Geometry check sheet. Reference: the model listing, model coordinates, mm. Face numbers are marked on the shaded views. A direction names the side the tool comes from. Round coordinates to 2 decimals unless told otherwise and drop trailing zeros. Order: outer loops, then holes, each group sorted by start corner. A loop starts at its lowest first (then second) coordinate and runs counter-clockwise, first axis right, second up.
(1) Material ranges on line 1 along Z through (x, y) = (-1.59, 16.65); line 2 along Z through (x, y) = (-1.2, 5.5); line 3 along Y through (x, z) = (-2.6, -7.75), recorded low to high.
(2) Set-up check for the marked faces 4, 5, 6, 7 and 8: record each of +Z, -Z, +X, -X, +Y, -Y from which the full face is reachable in a straight line by a thin tool's end or side.
(3) Go/stop test with flat-tipped pins: pin 1 (1.4 mm diameter, centred on x = -1.59, z = -8.1, fed in from -Y); pin 2 (3 mm diameter, centred on y = 11.25, z = 1.49, fed in from -X); pin 3 (1 mm diameter, centred on x = -1.5, y = 13, fed in from +Z). Record where each tip stops, or that it passes through.
(4) Release check for a two-part mould opening along Z. For the marked faces 1, 2 and 3 record: +Z half, -Z half, draft (parallel to the pull), parting line (faces both ways), or undercut.
(5) Sectioned sample at A-A (y = -18). Record the boundary of the cut face in (x, z).
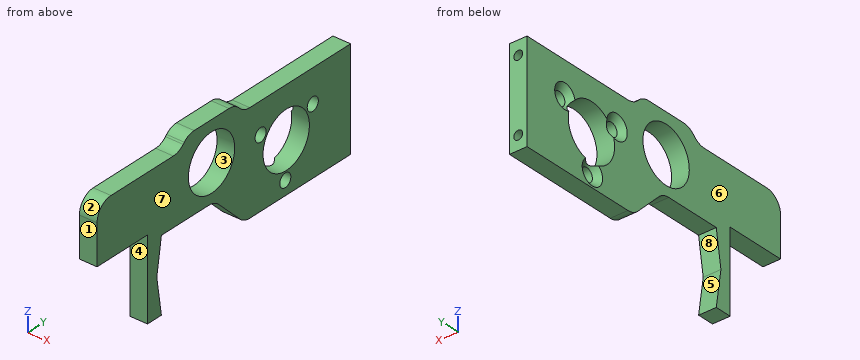
from build123d import *

# Parameters (mm, degrees)
BOSS_EXTRUDE1_DEPTH                             = 3.18
SKETCH2_4_OUTSIDE_W                             = 40.858
SKETCH2_4_OUTSIDE_H                             = 68.888
SKETCH2_4_OUTSIDE_R                             = 5
CUT_EXTRUDE2_DEPTH                              = 3.18
FILLET6_R                                       = 3
M2X0_4_TAPPED_HOLE1_D                           = 1.6
M2X0_4_TAPPED_HOLE1_DEPTH                       = 5.519311505
M2X0_4_TAPPED_HOLE1_TIP                         = 0.480688495
CUT_EXTRUDE3_REACH                              = 40.129
SKETCH7_R                                       = 1
CSK_FOR_M2_FLAT_HEAD_MACHINE_SCREW1_D           = 2.4
CSK_FOR_M2_FLAT_HEAD_MACHINE_SCREW1_DEPTH       = 3.18
CSK_FOR_M2_FLAT_HEAD_MACHINE_SCREW1_CSINK_D     = 4.4
CSK_FOR_M2_FLAT_HEAD_MACHINE_SCREW1_CSINK_ANGLE = 90


with BuildPart() as part:
    # Sketch2 → Boss-Extrude1 (new body)
    with BuildSketch(Plane(origin=(0, 0, 0), x_dir=(0, 0, -1), z_dir=(1, 0, 0))):
        Polygon((-7.39959254, 19.413571875), (10.60040746, 19.413571875), (10.60040746, -3.586428125), (4.27040746, -9.916428125), (4.27040746, -21.406428125), (10.625315102, -22.406428125), (17.27040746, -21.406428125), (17.27040746, -24.406428125), (2.77040746, -24.406428125), (2.77040746, -35.286428125), (-7.39959254, -35.286428125), (-7.39959254, -17.586428125), (-9.39959254, -15.586428125), (-9.39959254, -5.586428125), (-7.39959254, -3.586428125), align=None)
    extrude(amount=-BOSS_EXTRUDE1_DEPTH)

    # Sketch2<4> outside → Cut-Extrude2 (cut)
    # profile 1 of 3: a face of its own
    with BuildSketch(Plane(origin=(0, 0, 0), x_dir=(0, 0, -1), z_dir=(1, 0, 0))):
        with Locations((3.935, -7.936)):
            Rectangle(SKETCH2_4_OUTSIDE_W, SKETCH2_4_OUTSIDE_H)
        Polygon((-7.39959254, 19.413571875), (10.60040746, 19.413571875), (10.60040746, -3.586428125), (4.27040746, -9.916428125), (4.27040746, -21.406428125), (10.625315102, -22.406428125), (17.27040746, -21.406428125), (17.27040746, -24.406428125), (2.77040746, -24.406428125), (2.77040746, -35.286428125), (-7.39959254, -35.286428125), (-7.39959254, -17.586428125), (-9.39959254, -15.586428125), (-9.39959254, -5.586428125), (-7.39959254, -3.586428125), align=None, mode=Mode.SUBTRACT)
    # profile 2 of 3: a face of its own
    with BuildSketch(Plane(origin=(0, 0, 0), x_dir=(0, 0, -1), z_dir=(1, 0, 0))):
        with Locations((-2.39959254, -10.586428125)):
            Circle(SKETCH2_4_OUTSIDE_R)
    # profile 3 of 3: a face of its own
    with BuildSketch(Plane(origin=(0, 0, 0), x_dir=(0, 0, -1), z_dir=(1, 0, 0))):
        with Locations((1.60040746, 5.524437773)):
            Circle(SKETCH2_4_OUTSIDE_R)
    extrude(amount=-CUT_EXTRUDE2_DEPTH, mode=Mode.SUBTRACT)

    # Fillet6
    fillet6_edges = [part.edges().sort_by_distance(p)[0] for p in [
        (-1.59, -3.586428125, 7.39959254),
        (-1.59, -5.586428125, 9.39959254),
        (-1.59, -15.586428125, 9.39959254),
        (-1.59, -17.586428125, 7.39959254),
        (-1.59, -35.286428125, 7.39959254),
        (-1.59, -9.916428125, -4.27040746),
        (-1.59, -3.586428125, -10.60040746),
    ]]
    fillet(fillet6_edges, radius=FILLET6_R)

    # M2x0.4 Tapped Hole1
    with Locations(Plane(origin=(0, 19.413571875, 0), x_dir=(1, 0, 0), z_dir=(0, 1, 0))):
        with Locations((-1.59, 8.10040746), (-1.59, -4.89959254)):
            Hole(M2X0_4_TAPPED_HOLE1_D / 2, depth=M2X0_4_TAPPED_HOLE1_DEPTH)
            with Locations((0, 0, -(M2X0_4_TAPPED_HOLE1_DEPTH + M2X0_4_TAPPED_HOLE1_TIP / 2))):  # 118° drill point
                Cone(0, M2X0_4_TAPPED_HOLE1_D / 2, M2X0_4_TAPPED_HOLE1_TIP, mode=Mode.SUBTRACT)

    # Sketch7 → Cut-Extrude3 (cut, up to next)
    with BuildSketch(Plane(origin=(0, 0, -3.18), x_dir=(0, 0, -1), z_dir=(1, 0, 0)), mode=Mode.PRIVATE) as cut_extrude3_sk1:
        with Locations((-4.67466251, 11.25391193)):
            Circle(SKETCH7_R)
    cut_extrude3_tool1 = extrude(cut_extrude3_sk1.sketch, amount=-CUT_EXTRUDE3_REACH, mode=Mode.PRIVATE) & part.part
    # Sketch7 → Cut-Extrude3 (cut, up to next)
    with BuildSketch(Plane(origin=(0, 0, -3.18), x_dir=(0, 0, -1), z_dir=(1, 0, 0)), mode=Mode.PRIVATE) as cut_extrude3_sk2:
        with Locations((4.896479829, 5.325738996)):
            Circle(SKETCH7_R)
    cut_extrude3_tool2 = extrude(cut_extrude3_sk2.sketch, amount=-CUT_EXTRUDE3_REACH, mode=Mode.PRIVATE) & part.part
    # Sketch7 → Cut-Extrude3 (cut, up to next)
    with BuildSketch(Plane(origin=(0, 0, -3.18), x_dir=(0, 0, -1), z_dir=(1, 0, 0)), mode=Mode.PRIVATE) as cut_extrude3_sk3:
        with Locations((-5.023039699, 0.000973054)):
            Circle(SKETCH7_R)
    cut_extrude3_tool3 = extrude(cut_extrude3_sk3.sketch, amount=-CUT_EXTRUDE3_REACH, mode=Mode.PRIVATE) & part.part
    add(cut_extrude3_tool1.solids().sort_by_distance((0, 11.253912, 1.494663))[0], mode=Mode.SUBTRACT)
    add(cut_extrude3_tool2.solids().sort_by_distance((0, 5.325739, -8.07648))[0], mode=Mode.SUBTRACT)
    add(cut_extrude3_tool3.solids().sort_by_distance((0, 0.000973, 1.84304))[0], mode=Mode.SUBTRACT)

    # CSK for M2 Flat Head Machine Screw1
    with Locations(Plane.ZY.offset(3.18)):
        with Locations((-8.076479829, 5.325738996), (1.49466251, 11.25391193), (1.843039699, 0.000973054)):
            CounterSinkHole(CSK_FOR_M2_FLAT_HEAD_MACHINE_SCREW1_D / 2, CSK_FOR_M2_FLAT_HEAD_MACHINE_SCREW1_CSINK_D / 2, depth=CSK_FOR_M2_FLAT_HEAD_MACHINE_SCREW1_DEPTH, counter_sink_angle=CSK_FOR_M2_FLAT_HEAD_MACHINE_SCREW1_CSINK_ANGLE)


solid = part.part
Answer below:
1. line 1: z = -10.6 to -8.9, -7.3 to 4.1, 5.7 to 7.4
1. line 2: z = -10.6 to -9.26, -6.89 to -6.6, 3.4 to 7.4
1. line 3: y = -24.41 to -21.95, -6.44 to 3.74, 6.91 to 19.41
2. face 4: -Z, +X, -X, -Y
2. face 5: +X, -X, +Y
2. face 6: +Z, -Z, -X, +Y, -Y
2. face 7: +Z, -Z, +X, +Y, -Y
2. face 8: +X, -X
3. pin 1: stops at y = -24.41
3. pin 2: stops at x = -2.49
3. pin 3: stops at z = 7.4
4. face 1: draft
4. face 2: +Z half
4. face 3: undercut
5. outline: (-3.18, -4.27) - (0, -4.27) - (0, 7.52) - (-3.18, 7.52) - close
